from build123d import *

# Parameters (mm, degrees)
BOSS_EXTRUDE1_DEPTH     = 25
SKETCH2_R               = 15.25
BOSS_EXTRUDE2_DEPTH     = 144
SKETCH3_R               = 20
BOSS_EXTRUDE3_DEPTH     = 72
SKETCH4_R               = 9
BOSS_EXTRUDE4_DEPTH     = 26
CUT_EXTRUDE1_DEPTH      = 180.905530765
CUT_EXTRUDE1_DEPTH_BACK = 180.905530765
SKETCH5_R               = 4
SKETCH6_R               = 10
BOSS_EXTRUDE5_DEPTH     = 26
CUT_EXTRUDE2_DEPTH      = 205.523837242
CUT_EXTRUDE2_DEPTH_BACK = 205.523837242
SKETCH7_R               = 4


with BuildPart() as part:
    # Sketch1 → Boss-Extrude1 (new body)
    with BuildSketch(Plane(origin=(0, 0, 0), x_dir=(1, 0, 0), z_dir=(0, 1, 0))):
        with BuildLine():
            Line((-16, -24), (16, -24))
            Line((16, -24), (21, -19))
            Line((21, -19), (21, 37))
            ThreePointArc((21, 37), (0, 58), (-21, 37))
            Line((-21, 37), (-21, -19))
            Line((-21, -19), (-16, -24))
        make_face()
    extrude(amount=BOSS_EXTRUDE1_DEPTH)

    # Sketch2 → Boss-Extrude2 (add)
    with BuildSketch(Plane(origin=(0, 25, 0), x_dir=(1, 0, 0), z_dir=(0, 1, 0))):
        with Locations(Location((0, 0, 0), (0, 0, 270))):
            Circle(SKETCH2_R)
    extrude(amount=BOSS_EXTRUDE2_DEPTH)

    # Sketch3 → Boss-Extrude3 (add)
    with BuildSketch(Plane(origin=(0, 25, 0), x_dir=(1, 0, 0), z_dir=(0, 1, 0))):
        with Locations(Location((0, 37, 0), (0, 0, 270))):
            Circle(SKETCH3_R)
    extrude(amount=BOSS_EXTRUDE3_DEPTH)

    # Sketch4 → Boss-Extrude4 (add)
    with BuildSketch(Plane.XZ):
        with Locations(Location((0, 0, 0), (0, 0, 90))):
            Circle(SKETCH4_R)
    extrude(amount=BOSS_EXTRUDE4_DEPTH)

    # Sketch5 → Cut-Extrude1 (cut, two sides: drawn at the far end of the back side and taken through both)
    with BuildSketch(Plane(origin=(0, 0, 0), x_dir=(0, 0, -1), z_dir=(1, 0, 0)).offset(-CUT_EXTRUDE1_DEPTH_BACK)):
        with Locations((0, -20)):
            Circle(SKETCH5_R)
    extrude(amount=CUT_EXTRUDE1_DEPTH + CUT_EXTRUDE1_DEPTH_BACK, mode=Mode.SUBTRACT)

    # Sketch6 → Boss-Extrude5 (add)
    with BuildSketch(Plane(origin=(0, 169, 0), x_dir=(1, 0, 0), z_dir=(0, 1, 0))):
        with Locations(Location((0, 0, 0), (0, 0, 90))):
            Circle(SKETCH6_R)
    extrude(amount=BOSS_EXTRUDE5_DEPTH)

    # Sketch7 → Cut-Extrude2 (cut, two sides: drawn at the far end of the back side and taken through both)
    with BuildSketch(Plane(origin=(0, 0, 0), x_dir=(0, 0, -1), z_dir=(1, 0, 0)).offset(-CUT_EXTRUDE2_DEPTH_BACK)):
        with Locations((0, 189)):
            Circle(SKETCH7_R)
    extrude(amount=CUT_EXTRUDE2_DEPTH + CUT_EXTRUDE2_DEPTH_BACK, mode=Mode.SUBTRACT)


solid = part.part
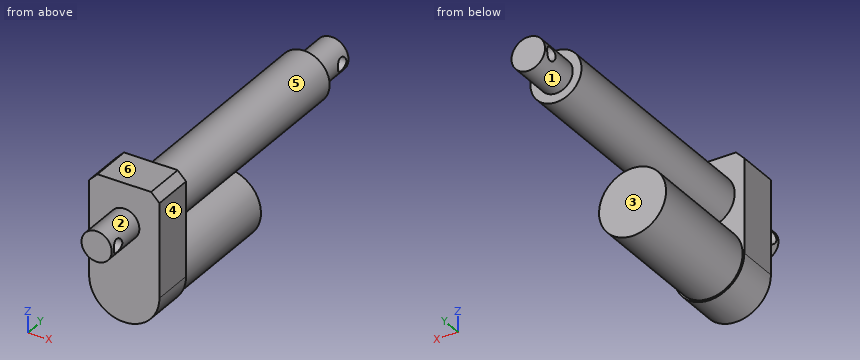
For this review, take the finished solid that the model builds, in its own axes (mm). Face numbers are marked on the shaded views. A direction names the side the tool comes from. Give positions to 0.01 mm unless a question says otherwise; leave off trailing zeros. Loops run counter-clockwise (first coordinate to the right, second up) from the corner with the lowest first, then second, coordinate; pieces in that order, holes last. Notation, with made-up numbers: M 22,-28.5 L 43,-28.5 A19 ccw 43,-9.5 Z; hole C 53,-39 d8. An arc over 180 degrees is marked long. Answer as a JSON object with one key per item and string values. Group by question number.
Q1. Add section A-A on x = 0. Give the boundary of the cut face in (y, z).
Q2. For probe 1 along Y at (x, z) = (-4, 0); probe 2 along Z at (x, y) = (0.5, 89); probe 3 along Y at (x, z) = (6.5, -41), list the stretches that pass through material, from the lowest coordinate up. Write a range as [from, to].
Q3. Add section D-D on z = 13. Give the boundary of the cut face in (x, y), and give its area (3 significant figures).
Q4. Add section C-C on y = 9.5. Give the boundary of the cut face in (x, z).
Q5. Insertion check: P1, Ø8, axis at y = 162.5, z = -5, coming from the -X side; P2, Ø12, axis at x = 11, y = 103.5, coming from the -Z side; P3, Ø2, axis at x = -3, z = -28.5, coming from the +Y side. Each pin has a flat end and moves straight along its axis. Give the tip position at first contact, or say it passes through.
Q6. Mouldability with a two-part tool opening along Z and no side actions: class the marked faces 4, 5 and 6 as +Z half, -Z half, draft (parallel to the pull), parting line (faces both ways), or undercut.
Q7. Tool access review of the marked faces 1, 2 and 3: name each direction out of +Z, -Z, +X, -X, +Y, -Y from which nothing blocks a thin tool from reaching the whole face with its end or side.
Q8. Add section B-B on z = 0. Give the boundary of the cut face in (x, y), and give its area (3 significant figures).
Checked values:
{
 "1": {"outline": "M -26,-9 L 0,-9 L 0,-58 L 25,-58 L 25,-57 L 97,-57 L 97,-17 L 25,-17 L 25,-15.25 L 169,-15.25 L 169,-10 L 195,-10 L 195,10 L 169,10 L 169,15.25 L 25,15.25 L 25,24 L 0,24 L 0,9 L -26,9 Z; hole C -20,0 d8; hole C 189,0 d8"},
 "2": {"probe 1": "[-26, -24], [-16, 185], [193, 195]", "probe 2": "[-56.99, -17.01], [-15.24, 15.24]", "probe 3": "[0, 97]"},
 "3": {"outline": "M -21,0 L 21,0 L 21,25 L 7.97,25 L 7.97,169 L -7.97,169 L -7.97,25 L -21,25 Z", "area": "3,350 mm²"},
 "4": {"outline": "M -21,-37 A21 ccw 21,-37 L 21,19 L 16,24 L -16,24 L -21,19 Z"},
 "5": {"P1": "x = -15.22", "P2": "z = -14.41", "P3": "y = 97"},
 "6": {"face 4": "draft", "face 5": "undercut", "face 6": "+Z half"},
 "7": {"face 1": "+Y", "face 2": "-Y", "face 3": "-Z, +X, -X, +Y"},
 "8": {"outline": "M -21,0 L -9,0 L -9,-16 L 9,-16 L 9,0 L 21,0 L 21,25 L 15.25,25 L 15.25,169 L 10,169 L 10,185 L -10,185 L -10,169 L -15.25,169 L -15.25,25 L -21,25 Z; M -10,193 L 10,193 L 10,195 L -10,195 Z; M -9,-26 L 9,-26 L 9,-24 L -9,-24 Z", "area": "6,130 mm²"}
}
